Work out the finished part from the listing and answer in its coordinate system (mm). A direction names the side the tool comes from. Round coordinates to 2 decimals unless told otherwise and drop trailing zeros. Loops run counter-clockwise (first coordinate to the right, second up) from the corner with the lowest first, then second, coordinate; pieces in that order, holes last. Notation, with made-up numbers: M -13,4.5 L 41,4.5 A28 ccw 41,39.5 Z; hole C -29,48.25 d1. An arc over 180 degrees is marked long. One line per item, written item: value.
```python
from build123d import *

# Parameters (mm, degrees)
SKETCH1_R                    = 31.75
SKETCH1_R_2                  = 19.05
BOSS_EXTRUDE1_DEPTH          = 12.7
SKETCH2_R                    = 31.75
SKETCH2_R_2                  = 19.05
BOSS_EXTRUDE2_DEPTH          = 38.1
SKETCH3_R                    = 25.4
CUT_EXTRUDE1_DEPTH           = 6.35
HOLE1_D                      = 9.525
HOLE1_DEPTH                  = 12.7
HOLE1_CBORE_D                = 15.875
HOLE1_CBORE_DEPTH            = 3.175
HOLE1_TIP                    = 2.861598698
F_3_8_0_375_DIAMETER_HOLE1_D = 9.525


with BuildPart() as part:
    # Sketch1 → Boss-Extrude1 (new body)
    # profile 1 of 3: a face of its own
    with BuildSketch(Plane(origin=(0, 0, 0), x_dir=(1, 0, 0), z_dir=(0, 1, 0))):
        with BuildLine():
            Line((-9.071428571, 30.426496408), (-49.892857143, 18.255897845))
            ThreePointArc((-49.892857143, 18.255897845), (-63.5, 0), (-49.892857143, -18.255897845))
            Line((-49.892857143, -18.255897845), (-9.071428571, -30.426496408))
            ThreePointArc((-9.071428571, -30.426496408), (-31.75, 0), (-9.071428571, 30.426496408))
        make_face()
    # profile 2 of 3: a face of its own
    with BuildSketch(Plane(origin=(0, 0, 0), x_dir=(1, 0, 0), z_dir=(0, 1, 0))):
        Circle(SKETCH1_R)
        with Locations(Location((0, 0, 0), (0, 0, 270))):
            Circle(SKETCH1_R_2, mode=Mode.SUBTRACT)
    # profile 3 of 3: a face of its own
    with BuildSketch(Plane(origin=(0, 0, 0), x_dir=(1, 0, 0), z_dir=(0, 1, 0))):
        with BuildLine():
            Line((49.892857143, 18.255897845), (9.071428571, 30.426496408))
            ThreePointArc((9.071428571, 30.426496408), (25.456633292, 18.974254173), (31.75, 0))
            ThreePointArc((31.75, 0), (25.456633292, -18.974254173), (9.071428571, -30.426496408))
            Line((9.071428571, -30.426496408), (49.892857143, -18.255897845))
            ThreePointArc((49.892857143, -18.255897845), (63.5, 0), (49.892857143, 18.255897845))
        make_face()
    extrude(amount=BOSS_EXTRUDE1_DEPTH)

    # Sketch2 → Boss-Extrude2 (add)
    with BuildSketch(Plane(origin=(0, 12.7, 0), x_dir=(1, 0, 0), z_dir=(0, 1, 0))):
        with Locations(Location((0, 0, 0), (0, 0, 106.601549599))):
            Circle(SKETCH2_R)
        with Locations(Location((0, 0, 0), (0, 0, 270))):
            Circle(SKETCH2_R_2, mode=Mode.SUBTRACT)
    extrude(amount=BOSS_EXTRUDE2_DEPTH)

    # Sketch3 → Cut-Extrude1 (cut)
    with BuildSketch(Plane(origin=(0, 50.8, 0), x_dir=(1, 0, 0), z_dir=(0, 1, 0))):
        with Locations(Location((0, 0, 0), (0, 0, 270))):
            Circle(SKETCH3_R)
    extrude(amount=-CUT_EXTRUDE1_DEPTH, mode=Mode.SUBTRACT)

    # Hole1
    with Locations(Plane(origin=(0, 12.7, 0), x_dir=(1, 0, 0), z_dir=(0, 1, 0))):
        with Locations((-44.45, 0), (44.45, 0)):
            CounterBoreHole(HOLE1_D / 2, HOLE1_CBORE_D / 2, HOLE1_CBORE_DEPTH, depth=HOLE1_DEPTH)
            with Locations((0, 0, -(HOLE1_DEPTH + HOLE1_TIP / 2))):  # 118° drill point
                Cone(0, HOLE1_D / 2, HOLE1_TIP, mode=Mode.SUBTRACT)

    # 3/8 (0.375) Diameter Hole1 (through all)
    with Locations(Plane(origin=(0, 31.75, -31.75), x_dir=(-1, 0, 0), z_dir=(0, 0, -1))):
        with Locations((0, 0)):
            Hole(F_3_8_0_375_DIAMETER_HOLE1_D / 2)


solid = part.part
```
1) Find the intervals of material crossed by probe 1 along X at (y, z) = (46, 0); probe 2 along X at (y, z) = (5.5, -2.5); probe 3 along Y at (x, z) = (-15, -16.5), in increasing order. Write a range as from..to.
Check values:
probe 1: -31.75..-25.4, 25.4..31.75
probe 2: -63.34..-48.5, -40.4..-18.89, 18.89..40.4, 48.5..63.34
probe 3: 0..44.45
2) For faces 1 (the face through (36.52, 11.13, -0.35)), 2 (the face through (63.497, 6.261, 0.342)), determine the directions among +Z, -Z, +X, -X, +Y, -Y from which every point of the face is accessible in a straight line to the end or side of a thin tool.
Check values:
face 1: +Y
face 2: +X, +Y, -Y
3) Find section D-D (x = 46). Give the vertices of the cut face in (y, z) (3 decimals), then the cut area to 3 significant figures.
Check values:
outline: M 0,-19.417 L 12.7,-19.417 L 12.7,-7.785 L 9.525,-7.785 L 9.525,-4.503 L 0,-4.503 Z; M 0,4.503 L 9.525,4.503 L 9.525,7.785 L 12.7,7.785 L 12.7,19.417 L 0,19.417 Z
area: 358 mm2
4) Find section B-B (z = 0). Give the number of separate pieces and of enclosed holes in the cut face, then the cut area to 3 significant figures.
Check values:
separate pieces: 4
enclosed holes: 0
area: 1,730 mm2
5) Each of these flat-tipped pins is pushed along its axis until it touches: pin 1 (1 mm diameter, centred on y = 25.5, z = -15.5, fed in from -X); pin 2 (10 mm diameter, centred on y = 42.5, z = 25, fed in from -X); pin 3 (5 mm diameter, centred on x = 48, z = 0.5, fed in from +Y) (3 decimals). Where does it stop, or does it pass through?
Check values:
pin 1: x = -27.98
pin 2: x = -24.66
pin 3: y = 9.525
6) Find section A-A (x = 0). Give the vertices of the cut face in (y, z), then the cut area to 3 significant figures.
Check values:
outline: M 0,-31.75 L 26.99,-31.75 L 26.99,-19.05 L 0,-19.05 Z; M 0,19.05 L 26.99,19.05 L 26.99,31.75 L 0,31.75 Z; M 36.51,-31.75 L 50.8,-31.75 L 50.8,-25.4 L 44.45,-25.4 L 44.45,-19.05 L 36.51,-19.05 Z; M 36.51,19.05 L 44.45,19.05 L 44.45,25.4 L 50.8,25.4 L 50.8,31.75 L 36.51,31.75 Z
area: 968 mm2
7) The mould has two halves that part along X. Classify faces 3 (the face through (-45, 9.525, 5)), 4 (the face through (29.196, 6.261, 24.426)), 5 (the face through (-52.38, 11.13, -0.35)), 6 (the face through (-63.497, 6.261, -0.342)): +X half, -X half, draft (parallel to the pull), parting line (faces both ways), or undercut.
Check values:
face 3: undercut
face 4: +X half
face 5: undercut
face 6: -X half
8) Find section C-C (y = 14.5). Give the vertices of the cut face in (x, z), then the cut area to 3 significant figures.
Check values:
outline: C 0,0 d63.5; hole C 0,0 d38.1
area: 2,030 mm2
